Print and shaded views of the part. All mm, measured from the part's lowest x, y and z. A direction names the side the tool comes from. Coordinates: 2 decimals unless noted, no trailing zeros. Order: outer loops, then holes, each group sorted by start corner. A loop starts at its lowest first (then second) coordinate and runs counter-clockwise, first axis right, second up. Notation, with made-up numbers: (42.25, -13.5) -> (80.25, -13.5) arc R35 cw to (80.25, 20.5) -> close; hole circle Ø3 at (-37.75, -7). An arc over 180 degrees is marked (long way). Write item = value, one per line. Start each with the question number.
Q1. Cut at D-D, the plane x = 115. List the corners of the cut face in (y, z) (1 decimal).
Q2. Flat gauge pins, fed straight in: pin 1 (10 mm diameter, centred on y = 63, z = 32.5, fed in from +X); pin 2 (12 mm diameter, centred on x = 124.5, y = 16, fed in from +Z). Where does each tip first touch, or does it go through?
Q3. 3-axis set-ups, long thin cutter, end or side, ignore diameter. For the marked faces 5, 6 and 7: which of +Z, -Z, +X, -X, +Y, -Y reach the whole face in a straight line?
Q4. Cut at C-C, the plane y = 40. List the corners of the cut face in (x, z).
Q5. Wall check: line 1 (Z direction, x = 127.5, y = 61); line 2 (X direction, y = 60.5, z = 37.5); line 3 (X direction, y = 59, z = 12) (1 decimal). Give the ranges that are in metal, low to high. Write a range as from..to.
Q6. Cut at B-B, the plane z = 19.5. List the corners of the cut face in (x, y), plus the area to 3 significant figures.
Q7. Cut at A-A, the plane y = 70.5. List the corners of the cut face in (x, z) (1 decimal).
Q8. Mould opens along X. For the marked faces 1, 2, 3 and 4 say: +X half, -X half, draft (parallel to the pull), parting line (faces both ways), or undercut.
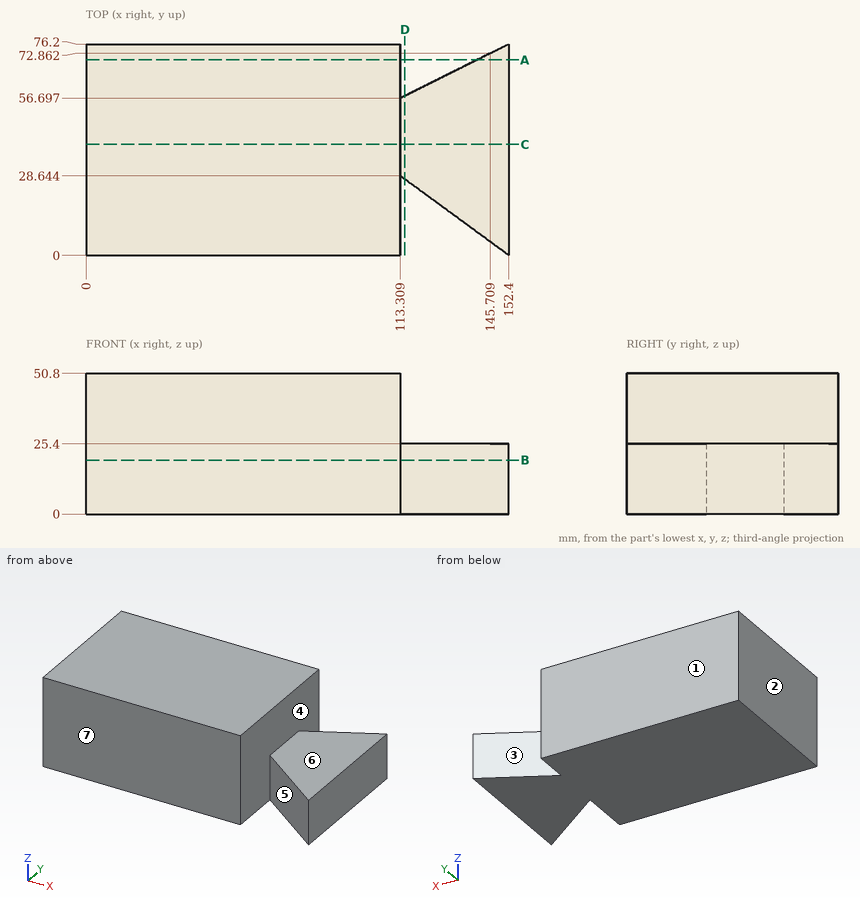
Here are the results:
q1.outline = (27.4, 0) -> (57.5, 0) -> (57.5, 25.4) -> (27.4, 25.4) -> close
q2.pin_1 = 113.31
q2.pin_2 = 25.4
q3.face_5 = +Z, -Z, -Y
q3.face_6 = +Z, +X, +Y, -Y
q3.face_7 = +Z, -Z, +X, -X, -Y
q4.outline = (0, 0) -> (152.4, 0) -> (152.4, 25.4) -> (113.31, 25.4) -> (113.31, 50.8) -> (0, 50.8) -> close
q5.line_1 = 0..25.4
q5.line_2 = 0..113.31
q5.line_3 = 0..113.3, 117.9..152.4
q6.outline = (0, 0) -> (113.31, 0) -> (113.31, 28.64) -> (152.4, 0) -> (152.4, 76.2) -> (113.31, 56.7) -> (113.31, 76.2) -> (0, 76.2) -> close
q6.area = 10,700 mm²
q7.outline = (0, 0) -> (113.3, 0) -> (113.3, 50.8) -> (0, 50.8) -> close; (141, 0) -> (152.4, 0) -> (152.4, 25.4) -> (141, 25.4) -> close
q8.face_1 = draft
q8.face_2 = -X half
q8.face_3 = undercut
q8.face_4 = undercut
